Part model, mm, in its own coordinate system. Round coordinates to 2 decimals unless told otherwise and drop trailing zeros. Write each loop counter-clockwise with the first axis right and the second up, starting at its lowest first coordinate (ties: lowest second). Pieces come first, ordered by that corner, then holes. Notation, with made-up numbers: M -36.5,-16 L 21.5,-16 A12 ccw 21.5,-2 Z; hole C 62.5,54.25 d5. An arc over 180 degrees is marked long. Use one line per item in the form item = value. Start each with the question number.
Item 1: Flat gauge pins, fed straight in: pin 1 Ø10 at (x, y) = (244, 13.5) entering from -Z; pin 2 Ø9.5 at (x, z) = (185.5, 11) entering from +Y; pin 3 Ø3 at (x, y) = (168.5, 15) entering from -Z. Where does each tip first touch, or does it go through?
Item 2: Cut at D-D, the plane x = 262. Give the cut face in (y, z) (3 decimals).
Item 3: Cut at A-A, the plane y = 14.5. Give the cut face in (x, z) (3 decimals), then the cut area to 3 significant figures.
Item 4: Cut at B-B, the plane z = 217. Give the cut face in (x, y) (3 decimals).
Item 5: Probe L1, parallel to Z at x = 198.5, y = 13.75; L2, parallel to Z at x = 320, y = 12; L3, parallel to X at y = 14, z = 218 (3 decimals). List the from-to ranges inside material, lowest first.
Item 6: Cut at C-C, the plane x = 152. Give the cut face in (y, z) (3 decimals), then the cut area to 3 significant figures.
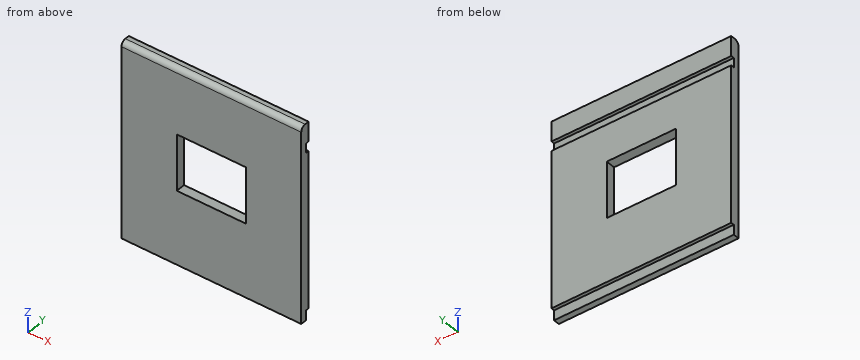
from build123d import *

# Parameters (mm, degrees)
SKETCH1_W           = 346.7
SKETCH1_H           = 376.55000001
BOSS_EXTRUDE1_DEPTH = 18
SKETCH2_W           = 346.7
SKETCH2_H           = 18
CUT_EXTRUDE1_DEPTH  = 6.35
SKETCH3_W           = 133.35
SKETCH3_H           = 107.95
CUT_EXTRUDE3_DEPTH  = 19
FILLET1_R           = 9.525
SKETCH6_W           = 346.7
SKETCH6_H           = 19.05
CUT_EXTRUDE4_DEPTH  = 6.35


with BuildPart() as part:
    # Sketch1 → Boss-Extrude1 (new body)
    with BuildSketch(Plane(origin=(0, 0, 0), x_dir=(1, 0, 0), z_dir=(0, 1, 0))):
        with Locations((173.35, -188.275000005)):
            Rectangle(SKETCH1_W, SKETCH1_H)
    extrude(amount=BOSS_EXTRUDE1_DEPTH)

    # Sketch2 → Cut-Extrude1 (cut)
    with BuildSketch(Plane(origin=(0, 18, 0), x_dir=(1, 0, 0), z_dir=(0, 1, 0))):
        with Locations((173.35, -329.45000001)):
            Rectangle(SKETCH2_W, SKETCH2_H)
    extrude(amount=-CUT_EXTRUDE1_DEPTH, mode=Mode.SUBTRACT)

    # Sketch3 → Cut-Extrude3 (cut, through all)
    with BuildSketch(Plane(origin=(0, 18, 0), x_dir=(1, 0, 0), z_dir=(0, 1, 0))):
        with Locations((173.35, -195.57500001)):
            Rectangle(SKETCH3_W, SKETCH3_H)
    extrude(amount=-CUT_EXTRUDE3_DEPTH, mode=Mode.SUBTRACT)

    # Fillet1
    fillet1_edges = [part.edges().sort_by_distance(p)[0] for p in [
        (173.35, 0, 376.55000001),
    ]]
    fillet(fillet1_edges, radius=FILLET1_R)

    # Sketch6 → Cut-Extrude4 (cut)
    with BuildSketch(Plane(origin=(0, 18, 0), x_dir=(1, 0, 0), z_dir=(0, 1, 0))):
        with Locations((173.35, -9.525)):
            Rectangle(SKETCH6_W, SKETCH6_H)
    extrude(amount=-CUT_EXTRUDE4_DEPTH, mode=Mode.SUBTRACT)


solid = part.part
Model answer:
q1.pin_1 = 0
q1.pin_2 = 11.65
q1.pin_3 = 19.05
q2.outline = M 0,0 L 11.65,0 L 11.65,19.05 L 18,19.05 L 18,320.45 L 11.65,320.45 L 11.65,338.45 L 18,338.45 L 18,376.55 L 9.525,376.55 A9.525 ccw 0,367.025 Z
q3.outline = M 0,19.05 L 346.7,19.05 L 346.7,320.45 L 0,320.45 Z; M 0,338.45 L 346.7,338.45 L 346.7,376.55 L 0,376.55 Z; hole M 106.675,141.6 L 240.025,141.6 L 240.025,249.55 L 106.675,249.55 Z
q3.area = 103,000 mm²
q4.outline = M 0,0 L 106.675,0 L 106.675,18 L 0,18 Z; M 240.025,0 L 346.7,0 L 346.7,18 L 240.025,18 Z
q5.L1 = 19.05 to 141.6, 249.55 to 320.45, 338.45 to 376.55
q5.L2 = 19.05 to 320.45, 338.45 to 376.55
q5.L3 = 0 to 106.675, 240.025 to 346.7
q6.outline = M 0,0 L 11.65,0 L 11.65,19.05 L 18,19.05 L 18,141.6 L 0,141.6 Z; M 0,249.55 L 18,249.55 L 18,320.45 L 11.65,320.45 L 11.65,338.45 L 18,338.45 L 18,376.55 L 9.525,376.55 A9.525 ccw 0,367.025 Z
q6.area = 4,580 mm²
